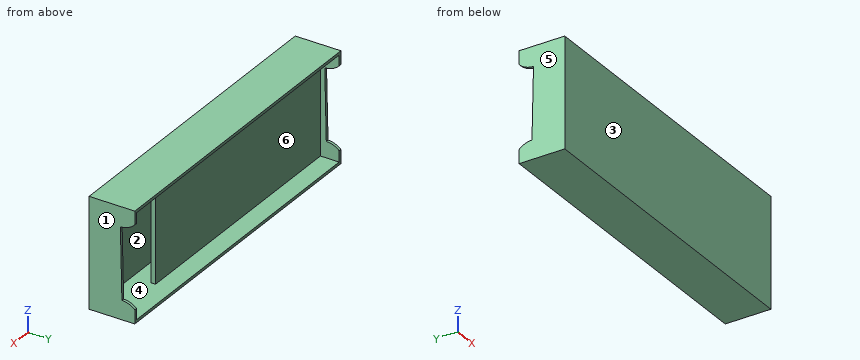
```python
from build123d import *

# Parameters (mm, degrees)
SKETCH1_W           = 175
SKETCH1_H           = 60
BOSS_EXTRUDE1_DEPTH = 25
SKETCH2_W           = 172.037419054
SKETCH2_H           = 56.878309912
CUT_EXTRUDE2_DEPTH  = 23
CUT_EXTRUDE4_DEPTH  = 180.30421077
SKETCH5_W           = 56.619672169
SKETCH5_H           = 2.543260903
BOSS_EXTRUDE2_DEPTH = 140


with BuildPart() as part:
    # Sketch1 → Boss-Extrude1 (new body)
    with BuildSketch(Plane(origin=(0, 0, 0), x_dir=(1, 0, 0), z_dir=(0, 1, 0))):
        Rectangle(SKETCH1_W, SKETCH1_H)
    extrude(amount=BOSS_EXTRUDE1_DEPTH)

    # Sketch2 → Cut-Extrude2 (cut)
    with BuildSketch(Plane(origin=(0, 25, 0), x_dir=(1, 0, 0), z_dir=(0, 1, 0))):
        Rectangle(SKETCH2_W, SKETCH2_H)
    extrude(amount=-CUT_EXTRUDE2_DEPTH, mode=Mode.SUBTRACT)

    # Sketch3 → Cut-Extrude4 (cut, through all)
    with BuildSketch(Plane(origin=(87.5, 0, 0), x_dir=(0, 0, -1), z_dir=(1, 0, 0))):
        with BuildLine():
            ThreePointArc((-22.681609782, 25), (-20.139304377, 21.416181436), (-19.241971202, 17.114801954))
            Line((-19.241971202, 17.114801954), (19.672994279, 17.951296347))
            ThreePointArc((19.672994279, 17.951296347), (20.393002527, 21.739785058), (22.452628009, 25))
            Line((22.452628009, 25), (-22.681609782, 25))
        make_face()
    extrude(amount=-CUT_EXTRUDE4_DEPTH, mode=Mode.SUBTRACT)

    # Sketch5 → Boss-Extrude2 (add)
    with BuildSketch(Plane(origin=(-86.018709527, 0, 0), x_dir=(0, 0, -1), z_dir=(1, 0, 0))):
        with Locations((0.129318872, 13.450991009)):
            Rectangle(SKETCH5_W, SKETCH5_H)
    extrude(amount=BOSS_EXTRUDE2_DEPTH)


solid = part.part
```
Read the model definition and answer for the solid it produces. Units are mm, in the model's axes. Face numbers are marked on the shaded views. A direction names the side the tool comes from. Coordinates: 2 decimals unless noted, no trailing zeros. Write each loop counter-clockwise with the first axis right and the second up, starting at its lowest first coordinate (ties: lowest second). Pieces come first, ordered by that corner, then holes. Notation, with made-up numbers: (31, -37.75) - (39, -37.75) arc R28 cw to (39, 0.25) - close; hole circle Ø3 at (0.5, -17.75). An arc over 180 degrees is marked (long way). Answer as a JSON object with one key per item and string values. Group by question number.
1. Which of the six approach directions +Z, -Z, +X, -X, +Y, -Y give full straight-line access (tool end or side, diameter ignored) to the marked faces 4, 5 and 6?
2. A cutting plane is placed at A-A (y = 7.5). Determine the outline of the cut face in (x, z).
3. A cutting plane is placed at C-C (z = 25.5). Determine the outline of the cut face in (x, y), plus the area to 3 significant figures.
4. A cutting plane is placed at B-B (x = 0). Determine the outline of the cut face in (y, z), plus the area to 3 significant figures.
5. Each of these flat-tipped pins is pushed along its axis until it touches: P1, Ø11.5, axis at y = 18, z = 13, coming from the +X side; P2, Ø1, axis at x = 12, z = 16.5, coming from the +Y side. Where does it stop, or does it pass through?
6. The mould has two halves that part along Y. Classify the marked faces 1, 2 and 3: +Y half, -Y half, draft (parallel to the pull), parting line (faces both ways), or undercut.
7. A cutting plane is placed at D-D (y = 21.75). Determine the outline of the cut face in (x, z), plus the area to 3 significant figures.
8. Consider L1, parallel to Y at x = 16, z = 14; L2, parallel to Z at x = -2, y = 20; L3, parallel to X at y = 11.75, z = -7. Determine where each line is inside the solid, lowest interval first. Write a range as [from, to].
Worked out:
{
 "1": {"face 4": "none", "face 5": "+Z, -Z, -X, +Y, -Y", "face 6": "+Y"},
 "2": {"outline": "(-87.5, -30) - (87.5, -30) - (87.5, 30) - (-87.5, 30) - close; hole (-86.02, -28.44) - (86.02, -28.44) - (86.02, 28.44) - (-86.02, 28.44) - close"},
 "3": {"outline": "(-87.5, 0) - (87.5, 0) - (87.5, 25) - (86.02, 25) - (86.02, 2) - (-86.02, 2) - (-86.02, 12.18) - (53.98, 12.18) - (53.98, 14.72) - (-86.02, 14.72) - (-86.02, 25) - (-87.5, 25) - close", "area": "774 mm²"},
 "4": {"outline": "(0, -30) - (25, -30) - (25, -28.44) - (14.72, -28.44) - (14.72, 28.18) - (12.18, 28.18) - (12.18, -28.44) - (2, -28.44) - (2, 28.44) - (25, 28.44) - (25, 30) - (0, 30) - close", "area": "336 mm²"},
 "5": {"P1": "stops at x = 87.5", "P2": "stops at y = 14.72"},
 "6": {"face 1": "draft", "face 2": "undercut", "face 3": "-Y half"},
 "7": {"outline": "(-87.5, -30) - (87.5, -30) - (87.5, -20.4) - (86.02, -20.4) - (86.02, -28.44) - (-86.02, -28.44) - (-86.02, -20.4) - (-87.5, -20.4) - close; (-87.5, 20.29) - (-86.02, 20.29) - (-86.02, 28.44) - (86.02, 28.44) - (86.02, 20.29) - (87.5, 20.29) - (87.5, 30) - (-87.5, 30) - close", "area": "594 mm²"},
 "8": {"L1": "y = [0, 2], [12.18, 14.72]", "L2": "z = [-30, -28.44], [28.44, 30]", "L3": "x = [-87.5, -86.02], [86.02, 87.5]"}
}
